For this review, take the finished solid that the model builds, in its own axes (mm). Face numbers are marked on the shaded views. A direction names the side the tool comes from. Round coordinates to 2 decimals unless told otherwise and drop trailing zeros. Loops run counter-clockwise (first coordinate to the right, second up) from the corner with the lowest first, then second, coordinate; pieces in that order, holes last. Notation, with made-up numbers: (-35.5, 5) -> (9.5, 5) arc R11 cw to (9.5, 23) -> close; hole circle Ø1 at (7.25, 2). An arc over 180 degrees is marked (long way). Write each question's results on one line, items separated by ' | '.
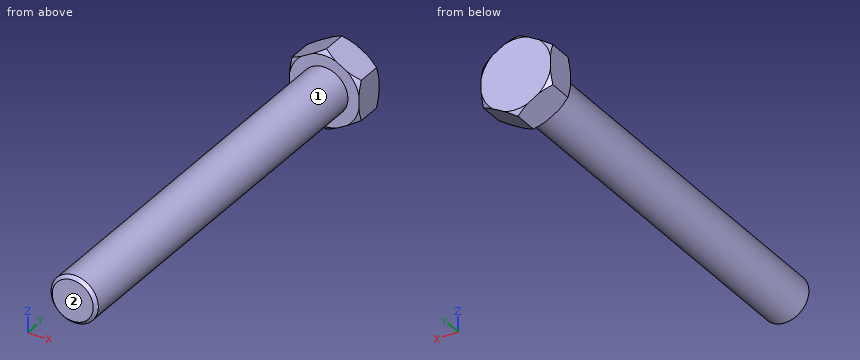
```python
from build123d import *

# Parameters (mm, degrees)
BOSS_EXTRUDE1_DEPTH = 10
SKETCH2_R           = 7.5
BOSS_EXTRUDE2_DEPTH = 126
CHAMFER1_SIZE       = 1
SCALE1_SCALE        = 0.25


with BuildPart() as part:
    # Sketch1 → Boss-Extrude1 (new body)
    with BuildSketch(Plane(origin=(0, 0, 0), x_dir=(1, 0, 0), z_dir=(0, 1, 0))):
        Polygon((11, -6.350852961), (11, 6.350852961), (0, 12.701705922), (-11, 6.350852961), (-11, -6.350852961), (0, -12.701705922), align=None)
    extrude(amount=-BOSS_EXTRUDE1_DEPTH)

    # Sketch2 → Boss-Extrude2 (add)
    with BuildSketch(Plane.XZ.offset(10)):
        with Locations(Location((0, 0, 0), (0, 0, 90))):
            Circle(SKETCH2_R)
    extrude(amount=BOSS_EXTRUDE2_DEPTH)

    # Sketch3 → Cut-Revolve1 (revolve, cut)
    with BuildSketch(Plane(origin=(0, 0, 0), x_dir=(0, 0, -1), z_dir=(1, 0, 0))):
        Polygon((-12.701705922, -1.2), (-11.201705922, 0), (-12.701705922, 0), align=None)
        Polygon((-12.701705922, -10), (-12.701705922, -8.8), (-11.201705922, -10), align=None)
    revolve(axis=Axis((0, 3.86627359, 0), (0, -1, 0)), mode=Mode.SUBTRACT)

    # Chamfer1
    chamfer1_edges = [part.edges().sort_by_distance(p)[0] for p in [
        (0, -136, -7.5),
    ]]
    chamfer(chamfer1_edges, length=CHAMFER1_SIZE)


with BuildPart() as part_1:
    # Scale1: scaled about (0, -62.210522466, 0)
    add(part.part.scale(SCALE1_SCALE).moved(Location((0, -46.65789185, 0))))


solid = part_1.part
```
1. Tool access review of the marked faces 1 and 2: name each direction out of +Z, -Z, +X, -X, +Y, -Y from which nothing blocks a thin tool from reaching the whole face with its end or side.
Values found:
face 1: -Y | face 2: +Z, -Z, +X, -X, -Y
2. To check wall thickness, follow probe 1 along Y at (x, z) = (2, -1.5); probe 2 along X at (y, z) = (-64, 0) (3 decimals); probe 3 along X at (y, z) = (-62, 1). State the ranges of each line that lie inside material, in increasing order.
Values found:
probe 1: y = -49.16 to -46.66 | probe 2: x = -1.875 to 1.875 | probe 3: x = -1.59 to 1.59
3. For pin 1 (1 mm diameter, centred on x = -0.5, y = -72.5, fed in from +Z) (3 decimals); pin 2 (1.5 mm diameter, centred on x = -0.5, y = -60, fed in from -Z) (3 decimals); pin 3 (2 mm diameter, centred on y = -54.5, z = 0.5, fed in from -X) (3 decimals), all flat-tipped, find the tip position at first contact; note any pin that passes through.
Values found:
pin 1: stops at z = 1.875 | pin 2: stops at z = -1.875 | pin 3: stops at x = -1.875
4. Consider section A-A (z = 0). State the section outline as (x, y) points (3 decimals).
Values found:
outline: (-2.75, -49.158) -> (-1.875, -49.158) -> (-1.875, -80.408) -> (-1.625, -80.658) -> (1.625, -80.658) -> (1.875, -80.408) -> (1.875, -49.158) -> (2.75, -49.158) -> (2.75, -46.658) -> (-2.75, -46.658) -> close
5. Consider section B-B (y = -73). State the section outline as (x, z) points (3 decimals), plus the area to 3 significant figures.
Values found:
outline: circle Ø3.75 at (0, 0) | area: 11.0 mm2
